from build123d import *

# Parameters (mm, degrees)
F1_DEPTH = 6.3
F3_D     = 4.4
F3_DEPTH = 6.223
F3_TIP   = 1.3218933619


with BuildPart() as f1:
    # F0 (on Top) → F1 (new body)
    with BuildSketch(Plane.XY):
        Polygon((4, 8.4201077782), (-4, 8.4201077782), (-7.5, 4.9201077782), (-7.5, -4), (-4, -7.5), (4, -7.5), (7.5, -4), (7.5, 4.9201077782), align=None)
    extrude(amount=F1_DEPTH)

    # F3
    with Locations(Plane(origin=(0, 0, 0), x_dir=(1, 0, 0), z_dir=(0, 0, -1))):
        with Locations((0, -1.7701077782)):
            Hole(F3_D / 2, depth=F3_DEPTH)
            with Locations((0, 0, -(F3_DEPTH + F3_TIP / 2))):  # 118° drill point
                Cone(0, F3_D / 2, F3_TIP, mode=Mode.SUBTRACT)


solid = f1.part
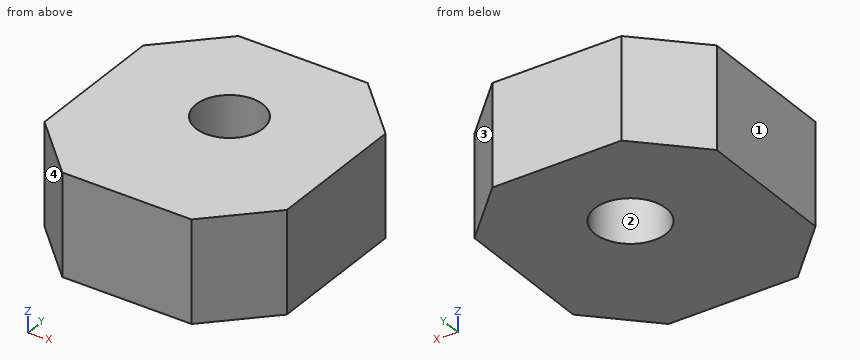
Geometry check sheet. Reference: the model listing, model coordinates, mm. Face numbers are marked on the shaded views. Give positions to 0.01 mm unless a question says otherwise; leave off trailing zeros. Loops run counter-clockwise (first coordinate to the right, second up) from the corner with the lowest first, then second, coordinate; pieces in that order, holes last. Notation, with made-up numbers: (33, 56.5) -> (88, 56.5) arc R33 ccw to (88, 86.5) -> close; hole circle Ø7 at (-28, 71). An arc over 180 degrees is marked (long way). Answer in a Markdown table with one row per item. Add a question column.
1) Cross-section at A-A on x = 0. Record the boundary of the cut face in (y, z).
2) Cross-section at B-B on z = 6. Record the boundary of the cut face in (x, y).
3) Gauge pin test, flat ends, axial feed: P1, Ø1, axis at x = 1, y = 7, coming from the -Z side; P2, Ø1, axis at x = -5, z = 2.5, coming from the -Y side. Record the tip position at first contact, or that the pin passes through.
4) Cross-section at D-D on y = 5.75. Record the boundary of the cut face in (x, z), and give its area (3 significant figures).
5) Material ranges on probe 1 along Y at (x, z) = (0, 2); probe 2 along Y at (x, z) = (-0.5, 5); probe 3 along X at (y, z) = (0, 0.75), recorded low to high. Write a range as from..to.
6) Cross-section at C-C on y = 7.5. Record the boundary of the cut face in (x, z).
7) Draft check along Y on the marked faces 1, 2, 3 and 4. Enter one of: pulls with the +Y half, pulls with the -Y half, needs draft (parallel to the pull), parting line crosses it, or undercut.
Outcome:
| question | item | result |
|---|---|---|
| 1 | outline | (-7.5, 0) -> (-0.43, 0) -> (-0.43, 6.22) -> (-0.3, 6.3) -> (-7.5, 6.3) -> close; (3.84, 6.3) -> (3.97, 6.22) -> (3.97, 0) -> (8.42, 0) -> (8.42, 6.3) -> close |
| 2 | outline | (-7.5, -4) -> (-4, -7.5) -> (4, -7.5) -> (7.5, -4) -> (7.5, 4.92) -> (4, 8.42) -> (-4, 8.42) -> (-7.5, 4.92) -> close; hole circle Ø4.4 at (0, 1.77) |
| 3 | P1 | stops at z = 0 |
| 3 | P2 | stops at y = -7 |
| 4 | outline | (-6.67, 0) -> (6.67, 0) -> (6.67, 6.3) -> (-6.67, 6.3) -> close |
| 4 | area | 84.0 mm^2 |
| 5 | probe 1 | y = -7.5..-0.43, 3.97..8.42 |
| 5 | probe 2 | y = -7.5..-0.37, 3.91..8.42 |
| 5 | probe 3 | x = -7.5..-1.31, 1.31..7.5 |
| 6 | outline | (-4.92, 0) -> (4.92, 0) -> (4.92, 6.3) -> (-4.92, 6.3) -> close |
| 7 | face 1 | needs draft |
| 7 | face 2 | undercut |
| 7 | face 3 | pulls with the +Y half |
| 7 | face 4 | pulls with the -Y half |
